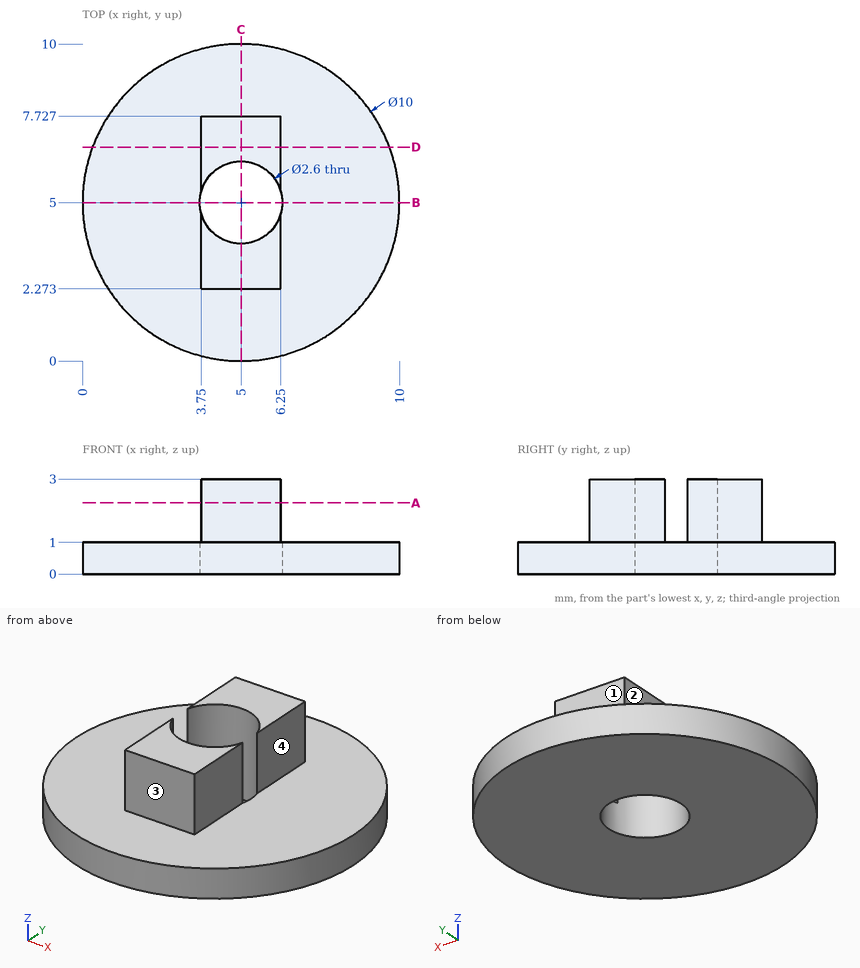
Study the drawing (mm; zero at the part's minimum x, y, z) and answer. A direction names the side the tool comes from. Round coordinates to 2 decimals unless told otherwise and drop trailing zeros. Write each loop counter-clockwise with the first axis right and the second up, starting at its lowest first coordinate (ties: lowest second). Pieces come first, ordered by that corner, then holes. Notation, with made-up numbers: (84.25, 3.25) - (117.25, 3.25) arc R27 cw to (117.25, 38.25) - close; hole circle Ø2 at (64.25, 53.5). An arc over 180 degrees is marked (long way). Return JSON: item names as keys, results as strings. Group by question number.
Q1. Each of these flat-tipped pins is pushed along its axis until it touches: pin 1 Ø1 at (y, z) = (3.5, 2) entering from -X; pin 2 Ø0.6 at (y, z) = (3.5, 1.5) entering from +X; pin 3 Ø0.6 at (x, z) = (4.5, 2) entering from -Y. Where does it stop, or does it pass through?
Q2. For the marked faces 1, 2, 3 and 4, determine the directions among +Z, -Z, +X, -X, +Y, -Y from which every point of the face is accessible in a straight line to the end or side of a thin tool.
Q3. The part is cut by section A-A on z = 2.25. Write down the section's boundary in (x, y).
Q4. The part is cut by section D-D on y = 6.75. Write down the section's boundary in (x, z).
Q5. Find the intervals of material crossed by L1, parallel to Y at x = 5, z = 0.8; L2, parallel to Y at x = 5, z = 2.7; L3, parallel to Z at x = 1, y = 3.75, in increasing order.
Q6. The part is cut by section B-B on y = 5. Write down the section's boundary in (x, z).
Q7. The part is cut by section C-C on x = 5. Write down the section's boundary in (y, z), then the cut area to 3 significant figures.
Solved:
{
 "1": {"pin 1": "x = 3.75", "pin 2": "x = 6.25", "pin 3": "y = 2.27"},
 "2": {"face 1": "+Z, +X, -X, +Y", "face 2": "+Z, -X, +Y, -Y", "face 3": "+Z, +X, -X, -Y", "face 4": "+Z, +X, +Y, -Y"},
 "3": {"outline": "(3.75, 2.27) - (6.25, 2.27) - (6.25, 4.64) arc R1.3 cw to (3.75, 4.64) - close; (3.75, 5.36) arc R1.3 cw to (6.25, 5.36) - (6.25, 7.73) - (3.75, 7.73) - close"},
 "4": {"outline": "(0.32, 0) - (9.68, 0) - (9.68, 1) - (6.25, 1) - (6.25, 3) - (3.75, 3) - (3.75, 1) - (0.32, 1) - close"},
 "5": {"L1": "0 to 3.7, 6.3 to 10", "L2": "2.27 to 3.7, 6.3 to 7.73", "L3": "0 to 1"},
 "6": {"outline": "(0, 0) - (3.7, 0) - (3.7, 1) - (0, 1) - close; (6.3, 0) - (10, 0) - (10, 1) - (6.3, 1) - close"},
 "7": {"outline": "(0, 0) - (3.7, 0) - (3.7, 3) - (2.27, 3) - (2.27, 1) - (0, 1) - close; (6.3, 0) - (10, 0) - (10, 1) - (7.73, 1) - (7.73, 3) - (6.3, 3) - close", "area": "13.1 mm²"}
}
